Geometry: final body of the model. Coordinates: model frame, mm. A direction names the side the tool comes from. Coordinates: 2 decimals unless noted, no trailing zeros. Write each loop counter-clockwise with the first axis right and the second up, starting at its lowest first coordinate (ties: lowest second). Pieces come first, ordered by that corner, then holes. Notation, with made-up numbers: (37, -26) - (82, -26) arc R12 cw to (82, -5) - close; hole circle Ø4 at (66, 14). An arc over 180 degrees is marked (long way). Answer as a JSON object with one key per item and string values. Group by question number.
Item 1: Set-up query: faces 1 (the flat face through (0, 2.5, 0)), 2 (the flat face through (0, 1, 3)), 3 (the flat face through (0, 0.7, 1)). Return all of +Z, -Z, +X, -X, +Y, -Y with unobstructed straight access to the full face (end or side cutting, diameter ignored); none if empty.
Item 2: Mould query, pull axis X, two halves, no side actions, for faces 4 (the flat face through (0, 1, -4.5)), 5 (the flat face through (3, 2, 0)), 6 (the cylindrical face through (-0.03, 0.85, 1.25)). Classes: pulls with the +X half, pulls with the -X half, needs draft (parallel to the pull), parting line crosses it, or undercut.
Item 3: Line query: line 1 along Y through (x, z) = (0.35, -1); line 2 along Z through (x, y) = (-2.4, 0.65); line 3 along Y through (x, z) = (-2.1, 4.75). Output: solid intervals per line, ascending. Write a range as from..to.
Item 4: Section A-A on x = -2.1. Return loops of the section in (y, z), and give its area (3 significant figures).
Item 5: Section C-C on y = 1.95. Return loops of the section in (x, z).
Item 6: First-contact query: pin 1 Ø1.8 at (x, z) = (1, 3) entering from -Y; pin 2 Ø1.5 at (x, y) = (1.5, 2) entering from +Z; pin 3 Ø0.8 at (x, z) = (0, 4) entering from -Y. Flat tips, straight axial feed; report the tip coordinate or a pass-through.
Item 7: Section B-B on z = 1.5. Return loops of the section in (x, y), and give its area (4 significant figures).
Item 8: Section D-D on x = 0. Return loops of the section in (y, z).
Autodesk Fusion 360 part; units mm, degrees
sketch "Sketch1" plane through (0, 0, 0) normal (0, 1, 0) x (1, 0, 0)
  line L0 (-3, 4.5) -> (3, 4.5)
  line L1 (3, 4.5) -> (3, -5.5)
  line L2 (3, -5.5) -> (-3, -5.5)
  line L3 (-3, -5.5) -> (-3, 4.5)
  line L4 (-1.25, -5.5) -> (-1.25, -2.5)
  arc A0 (1.25, -2.5) -> (-1.25, -2.5) centre (0, -2.5) ccw
  line L5 (1.25, -2.5) -> (1.25, -5.5)
  line L6 (-3, 3.5) -> (3, 3.5)
  line L7 (0, 0) -> (0, -2.5) construction
  dimension "d2" = 2.5
  dimension "d3" = 3
  dimension "d4" = 1
  dimension "d5" = 10
  dimension "d6" = 2.5
  dimension "d7" = 6
extrude "Extrude1" add sketch "Sketch1" along normal blind 2.5
extrude "Extrude2" cut sketch "Sketch1" along normal blind 0.7 contours L1 L2 L3 L4 A0 L5 L6 | L2 L4 A0 L5
extrude "Extrude3" cut sketch "Sketch1" along normal blind 1 contours L2 L4 A0 L5
hole "Hole1" at (0, 0, 0) direction (0, -1, 0) diameter 2.4 depth 5 tip angle 118
chamfer "Chamfer1" distance 0.5 angle 45 1 edges at (0, 0, -3.5)
chamfer "Chamfer2" distance 1 angle 45 1 edges at (0, 2.5, 5.5)
Checks:
{
 "1": {"face 1": "+Z, -Z, +X, -X, +Y", "face 2": "+Z, -Y", "face 3": "+Z, +X, -X, -Y"},
 "2": {"face 4": "needs draft", "face 5": "pulls with the +X half", "face 6": "undercut"},
 "3": {"line 1": "0.7..2.5", "line 2": "-4.5..-3.5", "line 3": "0.7..2.25"},
 "4": {"outline": "(0, -4.5) - (2.5, -4.5) - (2.5, 4.5) - (1.5, 5.5) - (0.7, 5.5) - (0.7, -3.5) - (0.5, -3.5) - (0, -4) - close", "area": "18.1 mm^2"},
 "5": {"outline": "(-3, -4.5) - (3, -4.5) - (3, 5.05) - (-3, 5.05) - close"},
 "6": {"pin 1": "y = 0.7", "pin 2": "z = 5.5", "pin 3": "y = 1"},
 "7": {"outline": "(-3, 0.7) - (-0.75, 0.7) - (-0.75, 1) - (0.75, 1) - (0.75, 0.7) - (3, 0.7) - (3, 2.5) - (-3, 2.5) - close", "area": "10.35 mm^2"},
 "8": {"outline": "(0, -4.5) - (2.5, -4.5) - (2.5, 4.5) - (1.5, 5.5) - (1, 5.5) - (1, 1.25) - (0.7, 1.25) - (0.7, -3.5) - (0.5, -3.5) - (0, -4) - close"}
}
